Part model, mm, in its own coordinate system. A direction names the side the tool comes from. Round coordinates to 2 decimals unless told otherwise and drop trailing zeros. Loops run counter-clockwise (first coordinate to the right, second up) from the corner with the lowest first, then second, coordinate; pieces in that order, holes last.
1) Drop flat-ended pins along their axis: P1, Ø5.5, axis at y = 176, z = 302, coming from the +X side; P2, Ø5, axis at y = 178.5, z = 148.5, coming from the +X side. Give the stop position or say it passes through.
2) Probe line 1 (Z direction, x = -390, y = 179.25); line 2 (X direction, y = 177, z = 147.5); line 3 (X direction, y = 175.5, z = 119.5). List the from-to ranges inside material, lowest first.
3) Band-saw the part on B-B, the plane y = 175. Write the cut outline in (x, z).
4) 3-axis set-ups, long thin cutter, end or side, ignore diameter. For faces 1 (the flat face through (-330.25, 175, 304)), 2 (the flat face through (-465.25, 178, 151)), 3 (the flat face through (-399, 179.064, 303)): which of +Z, -Z, +X, -X, +Y, -Y reach the whole face in a straight line?
5) Band-saw the part on A-A, the plane z = 274. Write the cut outline in (x, y), then the cut area to 3 significant figures.
from build123d import *

# Parameters (mm, degrees)
ESQUISSE1_W                         = 165.25
ESQUISSE1_H                         = 15.25
BOSS_EXTRU_1_DEPTH                  = 300
ESQUISSE3_W                         = 7
ESQUISSE3_H                         = 9
BOSS_EXTRU_4_DEPTH                  = 165.25
ENL_V_MAT_EXTRU_2_REACH             = 302
ENL_V_MAT_EXTRU_2_DIRECTION_2_REACH = 9
ESQUISSE4_W                         = 24
ESQUISSE4_H                         = 9
ENL_V_MAT_EXTRU_3_DEPTH             = 7


with BuildPart() as part:
    # Esquisse1 → Boss.-Extru.1 (new body)
    with BuildSketch(Plane.XY):
        with Locations((-382.625, 177.688864629)):
            Rectangle(ESQUISSE1_W, ESQUISSE1_H)
    extrude(amount=BOSS_EXTRU_1_DEPTH)

    # Esquisse3 → Boss.-Extru.4 (add)
    with BuildSketch(Plane.ZY.offset(465.25)):
        with Locations((303.5, 174.563864629)):
            Rectangle(ESQUISSE3_W, ESQUISSE3_H)
    extrude(amount=-BOSS_EXTRU_4_DEPTH)

    # Esquisse2 → Enlèv. mat.-Extru.2 (cut, up to next)
    with BuildSketch(Plane.XY.offset(300), mode=Mode.PRIVATE) as enl_v_mat_extru_2_sk1:
        Polygon((-300, 185.313864629), (-315.25, 170.063864629), (-300, 170.063864629), align=None)
    enl_v_mat_extru_2_tool1 = extrude(enl_v_mat_extru_2_sk1.sketch, amount=-ENL_V_MAT_EXTRU_2_REACH, mode=Mode.PRIVATE) & part.part
    add(enl_v_mat_extru_2_tool1.solids().sort_by_distance((-305.083333, 175.147198, 300))[0], mode=Mode.SUBTRACT)

    # Esquisse2 → Enlèv. mat.-Extru.2 direction 2 (cut, up to next)
    with BuildSketch(Plane.XY.offset(300), mode=Mode.PRIVATE) as enl_v_mat_extru_2_direction_2_sk1:
        Polygon((-300, 185.313864629), (-315.25, 170.063864629), (-300, 170.063864629), align=None)
    enl_v_mat_extru_2_direction_2_tool1 = extrude(enl_v_mat_extru_2_direction_2_sk1.sketch, amount=ENL_V_MAT_EXTRU_2_DIRECTION_2_REACH, mode=Mode.PRIVATE) & part.part
    add(enl_v_mat_extru_2_direction_2_tool1.solids().sort_by_distance((-305.083333, 175.147198, 300))[0], mode=Mode.SUBTRACT)

    # Esquisse4 → Enlèv. mat.-Extru.3 (cut)
    with BuildSketch(Plane.XY.offset(307)):
        with Locations((-318.25, 174.563864629)):
            Rectangle(ESQUISSE4_W, ESQUISSE4_H)
    extrude(amount=-ENL_V_MAT_EXTRU_3_DEPTH, mode=Mode.SUBTRACT)


solid = part.part
Reported:
1. P1: stops at x = -307.43
1. P2: stops at x = -304.31
2. line 1: z = 0 to 300
2. line 2: x = -465.25 to -308.31
2. line 3: x = -465.25 to -309.81
3. outline: (-465.25, 0) - (-310.31, 0) - (-310.31, 300) - (-330.25, 300) - (-330.25, 307) - (-465.25, 307) - close
4. face 1: +Z, +X, +Y, -Y
4. face 2: +Z, -Z, -X, +Y, -Y
4. face 3: +Z, +X, -X, +Y
5. outline: (-465.25, 170.06) - (-315.25, 170.06) - (-300, 185.31) - (-465.25, 185.31) - close
5. area: 2,400 mm2
